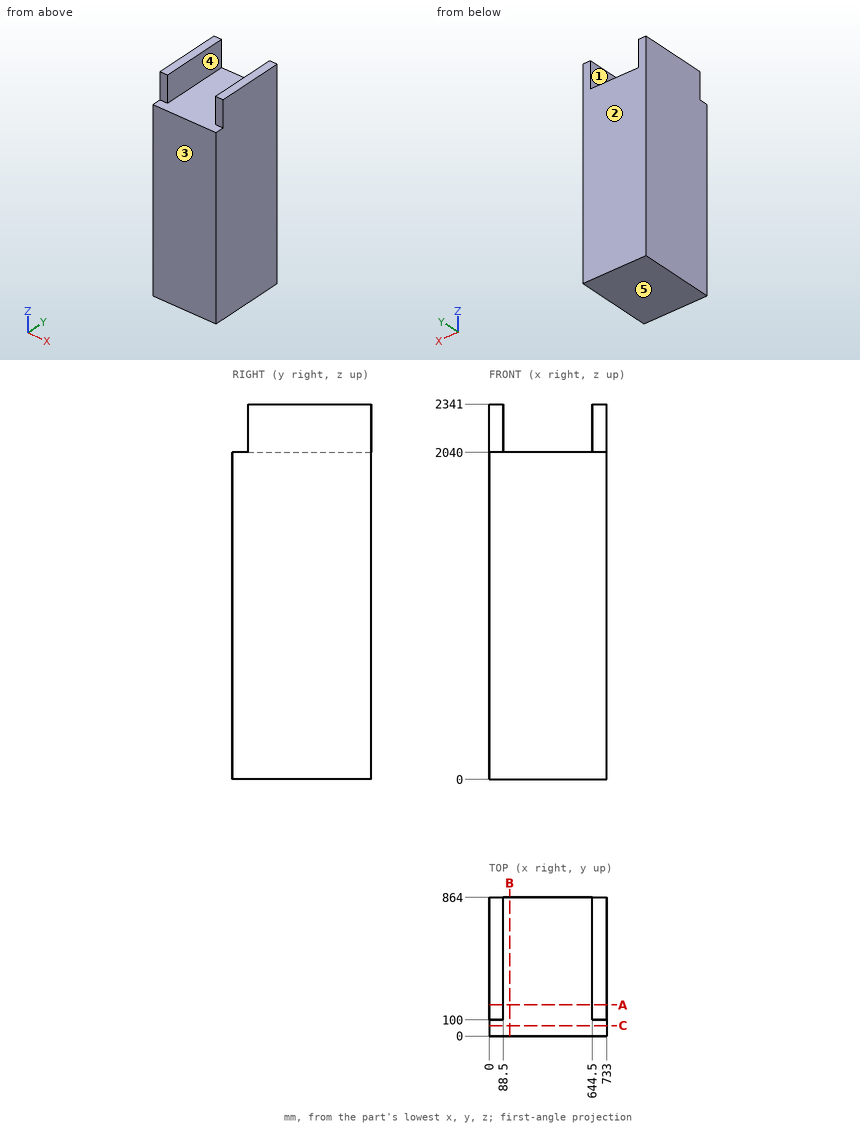
The figure shows three views and two pictorial views of one solid part (mm, origin at its lowest corner). Answer the questions. A direction names the side the tool comes from. Coordinates: 2 decimals unless noted, no trailing zeros. Order: outer loops, then holes, each group sorted by start corner. A loop starts at its lowest first (then second) coordinate and runs counter-clockwise, first axis right, second up. Notation, with made-up numbers: M 30,43 L 72,43 A16 ccw 72,47 Z; hole C 74,22 d8. An arc over 180 degrees is marked long. Use CSV: the item, a comma, the result in double quotes.
1) A flat-ended cylindrical pin translates along its axis: pin 1 Ø4 at (x, y) = (186.5, 722.5) entering from +Z. Find the tip coordinate at first contact, or state that the pin passes through.
Worked out:
pin 1,"stops at z = 2040"
2) For the marked faces 4 and 5, determine the directions among +Z, -Z, +X, -X, +Y, -Y from which every point of the face is accessible in a straight line to the end or side of a thin tool.
Worked out:
face 4,"+Z, +Y, -Y"
face 5,"-Z, +X, -X, +Y, -Y"
3) Consider line 1 (X direction, y = 587, z = 2079); line 2 (Z direction, x = 578, y = 262); line 3 (Y direction, x = 667.5, z = 2144.5). Determine where each line is inside the solid, lowest interval first. Write a range as [from, to].
Worked out:
line 1,"x = [0, 88.5], [644.5, 733]"
line 2,"z = [0, 2040]"
line 3,"y = [100, 864]"
4) Section C-C on y = 65 is taken. Write down the section's boundary in (x, z).
Worked out:
outline,"M 0,0 L 733,0 L 733,2040 L 0,2040 Z"
5) Section A-A on y = 194 is taken. Write down the section's boundary in (x, z).
Worked out:
outline,"M 0,0 L 733,0 L 733,2341 L 644.5,2341 L 644.5,2040 L 88.5,2040 L 88.5,2341 L 0,2341 Z"
6) Determine the mould class of the marked faces 1, 2 and 3 for opening direction Y: released by +Y, released by -Y, zero draft, split by the parting line, or undercut.
Worked out:
face 1,"zero draft"
face 2,"released by +Y"
face 3,"released by -Y"
7) Section B-B on x = 128 is taken. Write down the section's boundary in (y, z), plus the area to 3 significant figures.
Worked out:
outline,"M 0,0 L 864,0 L 864,2040 L 0,2040 Z"
area,"1,760,000 mm^2"
